Model file for the job. Use its own axes, mm. A direction names the side the tool comes from. Round coordinates to 2 decimals unless told otherwise and drop trailing zeros. Order: outer loops, then holes, each group sorted by start corner. A loop starts at its lowest first (then second) coordinate and runs counter-clockwise, first axis right, second up. Notation, with made-up numbers: M 46.5,80 L 61.5,80 A33 ccw 61.5,117 Z; hole C 82.25,1 d5. An arc over 180 degrees is marked long. Return JSON: item names as keys, results as strings. Group by question number.
Item 1: Slice it at B-B on x = 0. Write the cut outline in (y, z).
Item 2: Probe line 1 along Z through (x, y) = (0.5, 3); line 2 along X through (y, z) = (31, 0); line 3 along Z through (x, y) = (-11, 25). List the from-to ranges inside material, lowest first.
Item 3: Slice it at C-C on y = 14.5. Write the cut outline in (x, z).
Item 4: Pull direction Z, two halves, no side cores. Call faces 4 (the face through (14, 25.4, 4)), 5 (the face through (23.183, 18.783, 30.235)), 6 (the face through (-11.5, 0, -28)): pulls with the +Z half, pulls with the -Z half, needs draft (parallel to the pull), parting line crosses it, or undercut.
Item 5: Pin check, flat tips, straight feed: pin 1 Ø1 at (y, z) = (29.5, 13.5) entering from +X; pin 2 Ø3 at (y, z) = (16.5, 10) entering from +X; pin 3 Ø5 at (x, y) = (-18, 19) entering from +Z; pin 4 Ø22.5 at (x, z) = (0, 0) entering from -Y. Stop position of each tip, or through.
Item 6: Which spindle directions (+Z, -Z, +X, -X, +Y, -Y) get a long thin tool onto all of the face, cutting with end or side? Do faces 1 (the face through (-19.6, 31.8, -4.3)), 2 (the face through (29.78, 6.26, 3.91)), 3 (the face through (-5.38, 18.961, -12.975)). Say none if no direction does.
Item 7: Slice it at A-A on z = 0. Write the cut outline in (x, y), then the cut area to 3 significant figures.
Item 8: Slice it at D-D on x = 27. Write the cut outline in (y, z), then the cut area to 3 significant figures.
from build123d import *

# Parameters (mm, degrees)
SKETCH1_R           = 38.1
BOSS_EXTRUDE1_DEPTH = 38.1
SKETCH2_R           = 14.0462
CUT_EXTRUDE1_DEPTH  = 76.2
SKETCH3_R           = 20.066
CUT_EXTRUDE2_DEPTH  = 12.7
SKETCH4_R           = 30.0355
CUT_EXTRUDE3_DEPTH  = 12.7


with BuildPart() as part:
    # Sketch1 → Boss-Extrude1 (new body)
    with BuildSketch(Plane(origin=(0, 0, 0), x_dir=(1, 0, 0), z_dir=(0, 1, 0))):
        with Locations(Location((0, 0, 0), (0, 0, 90))):
            Circle(SKETCH1_R)
    extrude(amount=BOSS_EXTRUDE1_DEPTH)

    # Sketch2 → Cut-Extrude1 (cut)
    with BuildSketch(Plane.XZ):
        with Locations(Location((0, 0, 0), (0, 0, 270))):
            Circle(SKETCH2_R)
    extrude(amount=-CUT_EXTRUDE1_DEPTH, mode=Mode.SUBTRACT)

    # Sketch3 → Cut-Extrude2 (cut)
    with BuildSketch(Plane(origin=(0, 38.1, 0), x_dir=(1, 0, 0), z_dir=(0, 1, 0))):
        with Locations(Location((0, 0, 0), (0, 0, 270))):
            Circle(SKETCH3_R)
    extrude(amount=-CUT_EXTRUDE2_DEPTH, mode=Mode.SUBTRACT)

    # Sketch4 → Cut-Extrude3 (cut)
    with BuildSketch(Plane.XZ):
        with Locations(Location((0, 0, 0), (0, 0, 270))):
            Circle(SKETCH4_R)
    extrude(amount=-CUT_EXTRUDE3_DEPTH, mode=Mode.SUBTRACT)


solid = part.part
Output values:
{
 "1": {"outline": "M 0,-38.1 L 38.1,-38.1 L 38.1,-20.07 L 25.4,-20.07 L 25.4,-14.05 L 12.7,-14.05 L 12.7,-30.04 L 0,-30.04 Z; M 0,30.04 L 12.7,30.04 L 12.7,14.05 L 25.4,14.05 L 25.4,20.07 L 38.1,20.07 L 38.1,38.1 L 0,38.1 Z"},
 "2": {"line 1": "-38.1 to -30.03, 30.03 to 38.1", "line 2": "-38.1 to -20.07, 20.07 to 38.1", "line 3": "-36.48 to -8.73, 8.73 to 36.48"},
 "3": {"outline": "C 0,0 d76.2; hole C 0,0 d28.09"},
 "4": {"face 4": "undercut", "face 5": "parting line crosses it", "face 6": "needs draft"},
 "5": {"pin 1": "x = 35.81", "pin 2": "x = 37.14", "pin 3": "z = 34.8", "pin 4": "through"},
 "6": {"face 1": "+Y", "face 2": "-Y", "face 3": "+Y, -Y"},
 "7": {"outline": "M -38.1,0 L -30.04,0 L -30.04,12.7 L -14.05,12.7 L -14.05,25.4 L -20.07,25.4 L -20.07,38.1 L -38.1,38.1 Z; M 14.05,12.7 L 30.04,12.7 L 30.04,0 L 38.1,0 L 38.1,38.1 L 20.07,38.1 L 20.07,25.4 L 14.05,25.4 Z", "area": "1,270 mm²"},
 "8": {"outline": "M 0,-26.88 L 38.1,-26.88 L 38.1,26.88 L 0,26.88 L 0,13.16 L 12.7,13.16 L 12.7,-13.16 L 0,-13.16 Z", "area": "1,710 mm²"}
}
